Part model, mm, in its own coordinate system. Face numbers are marked on the shaded views. A direction names the side the tool comes from. Give positions to 0.01 mm unless a question says otherwise; leave off trailing zeros. Order: outer loops, then holes, each group sorted by start corner. A loop starts at its lowest first (then second) coordinate and runs counter-clockwise, first axis right, second up. Notation, with made-up numbers: M 36,-7 L 56,-7 A27 cw 56,23 Z; hole C 45.5,-5 d8. An arc over 180 degrees is marked long. Return JSON: item names as keys, results as strings.
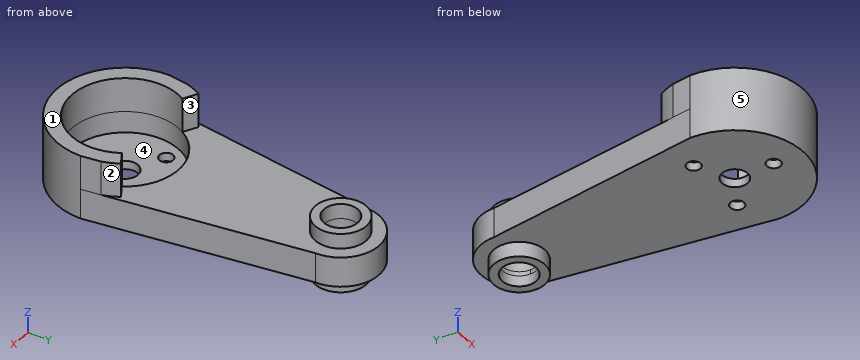
from build123d import *

# Parameters (mm, degrees)
BOSS_EXTRU_1_DEPTH      = 7
ESQUISSE2_R             = 3
ENL_V_MAT_EXTRU_1_DEPTH = 7
ESQUISSE3_R             = 1.6
ENL_V_MAT_EXTRU_2_DEPTH = 7
ESQUISSE5_R             = 12.5
ENL_V_MAT_EXTRU_5_DEPTH = 5
ESQUISSE16_R            = 6
ESQUISSE16_R_2          = 4
BOSS_EXTRU_5_DEPTH      = 3.5
BOSS_EXTRU_6_START      = 3.5
ESQUISSE17_R            = 6
ESQUISSE17_R_2          = 4
BOSS_EXTRU_6_DEPTH      = 3.5
BOSS_EXTRU_8_DEPTH      = 8
ESQUISSE19_R            = 4
ENL_V_MAT_EXTRU_6_DEPTH = 8


with BuildPart() as part:
    # Esquisse1 → Boss.-Extru.1 (new body)
    with BuildSketch(Plane.XY):
        with BuildLine():
            Line((9, 0), (16, -50))
            ThreePointArc((16, -50), (0, -66), (-16, -50))
            Line((-16, -50), (-9, 0))
            ThreePointArc((-9, 0), (0, 9), (9, 0))
        make_face()
    extrude(amount=BOSS_EXTRU_1_DEPTH)

    # Esquisse2 → Enlèv. mat.-Extru.1 (cut)
    with BuildSketch(Plane.XY.offset(7)):
        with Locations((0, -50)):
            Circle(ESQUISSE2_R)
    extrude(amount=-ENL_V_MAT_EXTRU_1_DEPTH, mode=Mode.SUBTRACT)

    # Esquisse3 → Enlèv. mat.-Extru.2 (cut)
    with BuildSketch(Plane.XY.offset(7)):
        with Locations((0, -59)):
            Circle(ESQUISSE3_R)
        with Locations((-7.794228634, -45.5)):
            Circle(ESQUISSE3_R)
        with Locations((7.794228634, -45.5)):
            Circle(ESQUISSE3_R)
    extrude(amount=-ENL_V_MAT_EXTRU_2_DEPTH, mode=Mode.SUBTRACT)

    # Esquisse5 → Enlèv. mat.-Extru.5 (cut)
    with BuildSketch(Plane.XY.offset(7)):
        with Locations((0, -50)):
            Circle(ESQUISSE5_R)
    extrude(amount=-ENL_V_MAT_EXTRU_5_DEPTH, mode=Mode.SUBTRACT)

    # Esquisse16 → Boss.-Extru.5 (add)
    with BuildSketch(Plane(origin=(0, 0, 0), x_dir=(-1, 0, 0), z_dir=(0, 0, -1))):
        Circle(ESQUISSE16_R)
        Circle(ESQUISSE16_R_2, mode=Mode.SUBTRACT)
    extrude(amount=BOSS_EXTRU_5_DEPTH)

    # Esquisse17 → Boss.-Extru.6 (add)
    with BuildSketch(Plane.XY.offset(7).offset(BOSS_EXTRU_6_START)):
        with Locations(Location((0, 0, 0), (0, 0, 180))):
            Circle(ESQUISSE17_R)
        with Locations(Location((0, 0, 0), (0, 0, 180))):
            Circle(ESQUISSE17_R_2, mode=Mode.SUBTRACT)
    extrude(amount=-BOSS_EXTRU_6_DEPTH)

    # Esquisse18 → Boss.-Extru.8 (add)
    with BuildSketch(Plane.XY.offset(7)):
        with BuildLine():
            Line((-10.825317547, -43.75), (-13.856406461, -42))
            ThreePointArc((-13.856406461, -42), (-14.731391476, -43.756114576), (-15.384856807, -45.606120047))
            Line((-15.384856807, -45.606120047), (-16, -50))
            ThreePointArc((-16, -50), (0, -66), (16, -50))
            Line((16, -50), (15.384856807, -45.606120047))
            ThreePointArc((15.384856807, -45.606120047), (14.731391476, -43.756114576), (13.856406461, -42))
            Line((13.856406461, -42), (10.825317547, -43.75))
            ThreePointArc((10.825317547, -43.75), (12.074072829, -46.764761936), (12.5, -50))
            ThreePointArc((12.5, -50), (-3.235238064, -62.074072829), (-10.825317547, -43.75))
        make_face()
    extrude(amount=BOSS_EXTRU_8_DEPTH)

    # Esquisse19 → Enlèv. mat.-Extru.6 (cut)
    with BuildSketch(Plane.XY.offset(7)):
        Circle(ESQUISSE19_R)
    extrude(amount=-ENL_V_MAT_EXTRU_6_DEPTH, mode=Mode.SUBTRACT)


solid = part.part
Q1. Probe line 1 along Y through (x, z) = (0, 8.8); line 2 along X through (y, z) = (-50, 9.5); line 3 along Y through (x, z) = (0, 1.05). List the from-to ranges inside material, lowest first.
Established:
{"line 1": "y = -66 to -62.5, -6 to -4, 4 to 6", "line 2": "x = -16 to -12.5, 12.5 to 16", "line 3": "y = -66 to -60.6, -57.4 to -53, -47 to -4, 4 to 9"}
Q2. Band-saw the part on A-A (x = 0). Give the cut face in (y, z), then the cut area to 3 significant figures.
Established:
{"outline": "M -66,0 L -60.6,0 L -60.6,2 L -62.5,2 L -62.5,15 L -66,15 Z; M -57.4,0 L -53,0 L -53,2 L -57.4,2 Z; M -47,0 L -6,0 L -6,-3.5 L -4,-3.5 L -4,10.5 L -6,10.5 L -6,7 L -37.5,7 L -37.5,2 L -47,2 Z; M 4,-3.5 L 6,-3.5 L 6,0 L 9,0 L 9,7 L 6,7 L 6,10.5 L 4,10.5 Z", "area": "382 mm²"}
Q3. Two-plate mould, pull along Y, no slides. Class the marked faces 3, 4 and 5: +Y half, -Y half, draft (parallel to the pull), parting line (faces both ways), or undercut.
Established:
{"face 3": "+Y half", "face 4": "undercut", "face 5": "-Y half"}
Q4. Band-saw the part on D-D (y = 2.5). Give the cut face in (x, z), then the cut area to 3 significant figures.
Established:
{"outline": "M -8.65,0 L -5.45,0 L -5.45,-3.5 L -3.12,-3.5 L -3.12,10.5 L -5.45,10.5 L -5.45,7 L -8.65,7 Z; M 3.12,-3.5 L 5.45,-3.5 L 5.45,0 L 8.65,0 L 8.65,7 L 5.45,7 L 5.45,10.5 L 3.12,10.5 Z", "area": "110 mm²"}
Q5. Pin check, flat tips, straight feed: pin 1 (8 mm diameter, centred on x = 0, y = -50, fed in from -Z); pin 2 (5 mm diameter, centred on x = 0, y = 0, fed in from +Z); pin 3 (7.5 mm diameter, centred on x = -2.5, y = -53, fed in from +Z); pin 4 (9 mm diameter, centred on x = -2, y = -30, fed in from +Z). Stop position of each tip, or through.
Established:
{"pin 1": "stops at z = 0", "pin 2": "passes through", "pin 3": "stops at z = 2", "pin 4": "stops at z = 7"}
Q6. 3-axis set-ups, long thin cutter, end or side, ignore diameter. For the marked faces 1 and 2: which of +Z, -Z, +X, -X, +Y, -Y reach the whole face in a straight line?
Established:
{"face 1": "+Z, +X, -X, +Y, -Y", "face 2": "+Z, +X, +Y"}
Q7. Band-saw the part on B-B (z = 1). Give the cut face in (x, y), then the cut area to 3 significant figures.
Established:
{"outline": "M -16,-50 A16 ccw 16,-50 L 9,0 A9 ccw -9,0 Z; hole C -7.79,-45.5 d3.2; hole C 0,0 d8; hole C 0,-50 d6; hole C 0,-59 d3.2; hole C 7.79,-45.5 d3.2", "area": "1,680 mm²"}
Q8. Band-saw the part on C-C (z = 13.75). Give the cut face in (x, y), then the cut area to 3 significant figures.
Established:
{"outline": "M -16,-50 A16 ccw 16,-50 L 15.38,-45.61 A16 ccw 13.86,-42 L 10.83,-43.75 A12.5 cw long -10.83,-43.75 L -13.86,-42 A16 ccw -15.38,-45.61 Z", "area": "208 mm²"}
